Autodesk Inventor part; units mm, degrees
ref_plane "YZ Plane" through (0, 0, 0) normal (1, 0, 0) x (0, 1, 0)
ref_plane "XZ Plane" through (0, 0, 0) normal (0, 1, 0) x (-1, 0, 0)
ref_plane "XY Plane" through (0, 0, 0) normal (0, 0, 1) x (1, 0, 0)
sketch "Schizzo1" plane through (0, 0, 0) normal (0, 0, 1) x (1, 0, 0)
  line L0 (-152.5, 86) -> (-2.5, 86) construction
  line L1 (-152.5, 0) -> (-152.5, 86) construction
  line L2 (-2.5, 0) -> (-2.5, 86) construction
  circle A0 centre (-9.5, 81) radius 1.5
  circle A1 centre (-147.5, 81) radius 1.5
  circle A2 centre (-147.5, 17) radius 1.5
  line L3 (4, 95) -> (-161, 95)
  line L4 (-161, -24) -> (-133, -24)
  line L5 (-128, -19) -> (-128, -19)
  line L6 (-123, -14) -> (-100, -14)
  line L7 (-95, -19) -> (-95, -19)
  line L8 (-90, -24) -> (-67, -24)
  line L9 (-62, -19) -> (-62, -19)
  line L10 (-57, -14) -> (-34, -14)
  line L11 (-29, -19) -> (-29, -19)
  line L12 (-24, -24) -> (4, -24)
  arc A3 (-133, -24) -> (-128, -19) centre (-133, -19) ccw
  arc A4 (-123, -14) -> (-128, -19) centre (-123, -19) ccw
  arc A5 (-95, -19) -> (-100, -14) centre (-100, -19) ccw
  arc A6 (-95, -19) -> (-90, -24) centre (-90, -19) ccw
  arc A7 (-67, -24) -> (-62, -19) centre (-67, -19) ccw
  arc A8 (-57, -14) -> (-62, -19) centre (-57, -19) ccw
  arc A9 (-29, -19) -> (-34, -14) centre (-34, -19) ccw
  arc A10 (-29, -19) -> (-24, -24) centre (-24, -19) ccw
  arc A11 (-17, 81) -> (-9.5, 73.5) centre (-9.5, 81) ccw
  arc A12 (-147.5, 73.5) -> (-140, 81) centre (-147.5, 81) ccw
  arc A13 (-140.4901, 19.6667) -> (-147.5, 24.5) centre (-147.5, 17) ccw
  line L13 (-147.5, 73.5) -> (-147.5, 24.5)
  line L14 (-17, 81) -> (-140, 81)
  line L15 (-9.5, 10) -> (-126.4703, 10)
  arc A14 (-140.4901, 19.6667) -> (-126.4703, 10) centre (-126.4703, 25) ccw
  line L16 (-9.5, 10) -> (-9.5, 73.5)
  line L17 (-161, 95) -> (-161, -24)
  line L18 (4, 95) -> (4, -24)
  line L19 (-161, -4) -> (-150, -4)
  line L20 (-150, 0) -> (-150, -4)
  line L21 (-150, 0) -> (-161, 0)
  line L22 (-161, 0) -> (-161, -4)
  line L23 (-139, -4) -> (-128, -4)
  line L24 (-128, 0) -> (-128, -4)
  line L25 (-128, 0) -> (-139, 0)
  line L26 (-139, 0) -> (-139, -4)
  line L27 (-117, -4) -> (-106, -4)
  line L28 (-106, 0) -> (-106, -4)
  line L29 (-106, 0) -> (-117, 0)
  line L30 (-117, 0) -> (-117, -4)
  line L31 (-95, -4) -> (-84, -4)
  line L32 (-84, 0) -> (-84, -4)
  line L33 (-84, 0) -> (-95, 0)
  line L34 (-95, 0) -> (-95, -4)
  line L35 (-73, -4) -> (-62, -4)
  line L36 (-62, 0) -> (-62, -4)
  line L37 (-62, 0) -> (-73, 0)
  line L38 (-73, 0) -> (-73, -4)
  line L39 (-51, -4) -> (-40, -4)
  line L40 (-40, 0) -> (-40, -4)
  line L41 (-40, 0) -> (-51, 0)
  line L42 (-51, 0) -> (-51, -4)
  line L43 (-29, -4) -> (-18, -4)
  line L44 (-18, 0) -> (-18, -4)
  line L45 (-18, 0) -> (-29, 0)
  line L46 (-29, 0) -> (-29, -4)
  line L47 (-7, -4) -> (4, -4)
  line L48 (-7, 0) -> (-7, -4)
  line L49 (-147.5, 82.5) -> (-147.5, 79.5) construction
  line L50 (-149, 82.5) -> (-149, 79.5)
  line L51 (-146, 79.5) -> (-146, 82.5)
  arc A15 (-146, 82.5) -> (-149, 82.5) centre (-147.5, 82.5) ccw
  arc A16 (-149, 79.5) -> (-146, 79.5) centre (-147.5, 79.5) ccw
  line L52 (-9.5, 82.5) -> (-9.5, 79.5) construction
  line L53 (-11, 82.5) -> (-11, 79.5)
  line L54 (-8, 79.5) -> (-8, 82.5)
  arc A17 (-8, 82.5) -> (-11, 82.5) centre (-9.5, 82.5) ccw
  arc A18 (-11, 79.5) -> (-8, 79.5) centre (-9.5, 79.5) ccw
  line L55 (-147.5, 18.5) -> (-147.5, 15.5) construction
  line L56 (-149, 18.5) -> (-149, 15.5)
  line L57 (-146, 15.5) -> (-146, 18.5)
  arc A19 (-146, 18.5) -> (-149, 18.5) centre (-147.5, 18.5) ccw
  arc A20 (-149, 15.5) -> (-146, 15.5) centre (-147.5, 15.5) ccw
  line L58 (4, 0) -> (4, -4)
  line L59 (4, 0) -> (-7, 0)
  point P0 (-128, -24)
  point P1 (-128, -14)
  point P2 (-95, -14)
  point P3 (-95, -24)
  point P4 (-62, -24)
  point P5 (-62, -14)
  point P6 (-29, -14)
  point P7 (-29, -24)
  point P8 (-144.8074, 10)
  dimension "d0" = 165
  dimension "d9" = 33
  dimension "d10" = 10
  dimension "d11" = 33
  dimension "d12" = 10
  dimension "d13" = 33
  dimension "d14" = 10
  dimension "d15" = 33
  dimension "d16" = 5
  dimension "d21" = 15
extrude "Estrusione1" add sketch "Schizzo1" along normal blind 4 contours L18 L59 L48 L47 L12 A10 A9 L10 A8 A7 L8 A6 A5 L6 A4 A3 L4 L17 L19 L20 L21 L3
sketch "Schizzo2" plane through (0, 0, 4) normal (0, 0, 1) x (1, 0, 0)
  line L0 (-157, 85.5) -> (-161, 85.5)
  line L1 (-161, 85.5) -> (-161, 95)
  line L2 (-161, 95) -> (-157, 95)
  line L3 (-157, 95) -> (-157, 85.5)
  line L4 (-157, 66.5) -> (-161, 66.5)
  line L5 (-161, 66.5) -> (-161, 76)
  line L6 (-161, 76) -> (-157, 76)
  line L7 (-157, 76) -> (-157, 66.5)
  line L8 (-161, 57) -> (-157, 57)
  line L9 (-157, 57) -> (-157, 47.5)
  line L10 (-157, 47.5) -> (-161, 47.5)
  line L11 (-161, 47.5) -> (-161, 57)
  line L12 (-157, 28.5) -> (-161, 28.5)
  line L13 (-161, 28.5) -> (-161, 38)
  line L14 (-161, 38) -> (-157, 38)
  line L15 (-157, 38) -> (-157, 28.5)
  line L16 (-161, 19) -> (-157, 19)
  line L17 (-157, 19) -> (-157, 9.5)
  line L18 (-157, 9.5) -> (-161, 9.5)
  line L19 (-161, 9.5) -> (-161, 19)
  point P0 (0, 0)
extrude "Estrusione2" cut sketch "Schizzo2" against normal blind 4
fillet "Raccordo1" radius 15 1 edges at (4, 95, 2)
fillet "Raccordo2" radius 10 1 edges at (4, -24, 2)
sketch "Schizzo3" plane through (0, 0, 4) normal (0, 0, 1) x (1, 0, 0)
  line L0 (-14.15, 0) -> (-10.85, 0)
  line L1 (-146.15, 0) -> (-142.85, 0)
  line L2 (-144.5, 0) -> (-144.5, 7) construction
  line L3 (-144.5, 0) -> (-137.5, 0) construction
  line L4 (-12.5, 0) -> (-12.5, 7) construction
  circle A0 centre (-144.5, 7) radius 1.65
  circle A1 centre (-12.5, 7) radius 1.65
  line L5 (-157, 82.4) -> (-157, 79.1) construction
  line L6 (-157, 85.5) -> (-157, 95) construction
  line L7 (-157, 95) -> (-157, 85.5)
  line L8 (-157, 90.25) -> (-150, 90.25) construction
  circle A2 centre (-150, 90.25) radius 1.65
  line L9 (-157, -12.35) -> (-157, -15.65) construction
  line L10 (-157, -14) -> (-150, -14) construction
  circle A3 centre (-150, -14) radius 1.65
  point P0 (0, 0)
  dimension "d28" = 7
  dimension "d29" = 90
  dimension "d30" = 7
  dimension "d31" = 3.3
  dimension "d32" = 3.3
  dimension "d35" = 7
  dimension "d36" = 3.3
  dimension "d37" = 7
  dimension "d38" = 3.3
extrude "Estrusione3" cut sketch "Schizzo3" against normal blind 4
properties part number "LatoAlimentatore"
The model under review builds one solid part; all positions refer to its coordinate system, in mm. A direction names the side the tool comes from. Give positions to 0.01 mm unless a question says otherwise; leave off trailing zeros. Write each loop counter-clockwise with the first axis right and the second up, starting at its lowest first coordinate (ties: lowest second). Pieces come first, ordered by that corner, then holes. Notation, with made-up numbers: (86.5, 67.25) - (129.5, 67.25) arc R9 ccw to (129.5, 84.25) - close; hole circle Ø5 at (-21, 54.25). An arc over 180 degrees is marked (long way). Answer in a Markdown table with one row per item. Add a question column.
1. Insertion check: P1, Ø1.2, axis at x = -160, z = 2, coming from the +Y side; P2, Ø1.2, axis at y = 69.5, z = 2.5, coming from the -X side; P3, Ø1.2, axis at x = 0.5, z = 1.5, coming from the -Y side; P4, Ø1, axis at x = -16, y = -10, coming from the -Z side. Each pin has a flat end and moves straight along its axis. Give the tip position at first contact, or say it passes through.
2. Wall thickness on line 1 along Y through (x, z) = (-24, 0.4); line 2 along Y through (x, z) = (-45.5, 3.7); line 3 along X through (y, z) = (46.5, 0.4): over which ranges is each line inside the solid? List them lowest first. Write a range as [from, to].
3. We need section C-C on z = 3.4. State how many separate pieces and enclosed holes the cut face has, then the cut area to 3 significant figures.
4. Draft analysis for pull direction X (two halves, no side actions). For faces 1 (the flat face through (-161, 24, 2)), 2 (the flat face through (-159, 57, 2)), 3 (the flat face through (-46, -4, 2)), state which applies: +X half, -X half, draft (parallel to the pull), parting line (faces both ways), or undercut.
5. We need section B-B on x = -104. Write out the cut boundary in (y, z), then the cut area to 3 significant figures.
6. We need section A-A on y = 63. Write out the cut boundary in (x, z).
7. Tool access review of faces 4 (the flat face through (-90, -4, 2)), 5 (the flat face through (-157, 90, 2)), 6 (the flat face through (-157, 71, 2)): name each direction out of +Z, -Z, +X, -X, +Y, -Y from which nothing blocks a thin tool from reaching the whole face with its end or side.
Ans:
| question | item | result |
|---|---|---|
| 1 | P1 | stops at y = 85.5 |
| 1 | P2 | stops at x = -157 |
| 1 | P3 | stops at y = -22.07 |
| 1 | P4 | stops at z = 0 |
| 2 | line 1 | y = [-24, -4], [0, 10], [81, 95] |
| 2 | line 2 | y = [-14, -4], [0, 10], [81, 95] |
| 2 | line 3 | x = [-161, -147.5], [-9.5, 4] |
| 3 | separate pieces | 1 |
| 3 | enclosed holes | 14 |
| 3 | area | 8,700 mm^2 |
| 4 | face 1 | -X half |
| 4 | face 2 | draft |
| 4 | face 3 | undercut |
| 5 | outline | (-14, 0) - (10, 0) - (10, 4) - (-14, 4) - close; (81, 0) - (95, 0) - (95, 4) - (81, 4) - close |
| 5 | area | 152 mm^2 |
| 6 | outline | (-161, 0) - (-147.5, 0) - (-147.5, 4) - (-161, 4) - close; (-9.5, 0) - (4, 0) - (4, 4) - (-9.5, 4) - close |
| 7 | face 4 | +Z, -Z |
| 7 | face 5 | +Z, -Z, -X, +Y |
| 7 | face 6 | +Z, -Z, -X |
